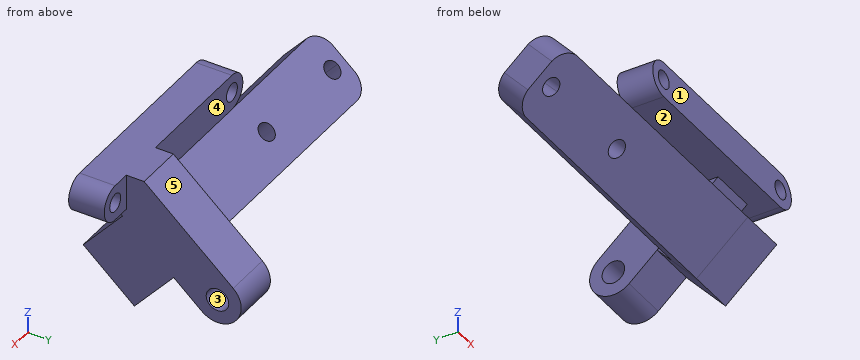
```python
from build123d import *

# Parameters (mm, degrees)
SKETCH_1_R          = 1.5
SKETCH_1_W          = 8
SKETCH_1_H          = 6
EXTRUDE_2_DEPTH     = 6
SKETCH_1_4_W        = 8
SKETCH_1_4_H        = 3
EXTRUDE_3_DEPTH     = 3
EXTRUDE_28_DEPTH    = 8
SKETCH_4_W          = 7.960549586
SKETCH_4_H          = 11.5
EXTRUDE_29_DEPTH    = 10
EXTRUDE_30_DEPTH    = 50
SKETCH_7_R          = 1.5
CUT_EXTRUDE_1_DEPTH = 10
SKETCH_8_R          = 1.9
CUT_EXTRUDE_2_DEPTH = 19


with BuildPart() as part:
    # Sketch 1 → Extrude 2 (new body)
    # profile 1 of 2: a face of its own
    with BuildSketch(Plane(origin=(0, 0, 0), x_dir=(1, 0, 0), z_dir=(0, 1, 0))):
        with BuildLine():
            Line((-38.676968887, 3), (-6.676968887, 3))
            ThreePointArc((-6.676968887, 3), (-3.676968887, 0), (-6.676968887, -3))
            Line((-6.676968887, -3), (-38.676968887, -3))
            ThreePointArc((-38.676968887, -3), (-41.676968887, 0), (-38.676968887, 3))
        make_face()
        with Locations(Location((-6.676968887, 0, 0), (0, 0, 270))):
            Circle(SKETCH_1_R, mode=Mode.SUBTRACT)
        with Locations(Location((-38.676968887, 0, 0), (0, 0, 270))):
            Circle(SKETCH_1_R, mode=Mode.SUBTRACT)
    # profile 2 of 2: a face of its own
    with BuildSketch(Plane(origin=(0, 0, 0), x_dir=(1, 0, 0), z_dir=(0, 1, 0))):
        with Locations((-13.722758256, 0)):
            Rectangle(SKETCH_1_W, SKETCH_1_H)
    extrude(amount=-EXTRUDE_2_DEPTH)

    # Sketch 1_4 → Extrude 3 (add)
    with BuildSketch(Plane(origin=(0, 0, 0), x_dir=(1, 0, 0), z_dir=(0, 1, 0))):
        with Locations((-13.722758256, -1.5)):
            Rectangle(SKETCH_1_4_W, SKETCH_1_4_H)
        with Locations((-13.722758256, 1.5)):
            Rectangle(SKETCH_1_4_W, SKETCH_1_4_H)
    extrude(amount=EXTRUDE_3_DEPTH)

    # Sketch 3 → Extrude 28 (add)
    with BuildSketch(Plane(origin=(-9.722758256, 0, 0), x_dir=(0, 0, -1), z_dir=(1, 0, 0))):
        with BuildLine():
            Line((3, -2.291502622), (16.228756555, 12.708497378))
            ThreePointArc((16.228756555, 12.708497378), (15.874507866, 18.354248689), (10.228756555, 18))
            Line((10.228756555, 18), (-3, 3))
            Line((-3, 3), (3, -2.291502622))
        make_face()
    extrude(amount=-EXTRUDE_28_DEPTH)

    # Sketch 4 → Extrude 29 (add)
    with BuildSketch(Plane(origin=(0, -2.49076751, -2.824264888), x_dir=(-1, 0, 0), z_dir=(0, -0.6614378277661491, -0.7499999999999987))):
        with Locations((13.703033049, 8.211179299)):
            Rectangle(SKETCH_4_W, SKETCH_4_H)
    extrude(amount=EXTRUDE_29_DEPTH)

    # Sketch 6 → Extrude 30 (add)
    with BuildSketch(Plane.ZY.offset(17.683307842)):
        Polygon((-19.558716996, 1.365738687), (-11.952181977, -7.259261313), (-7.452181977, -3.290634347), (-15.058716996, 5.334365653), align=None)
    extrude(amount=EXTRUDE_30_DEPTH)

    # Sketch 7 → Cut-Extrude 1 (cut)
    with BuildSketch(Plane(origin=(0, -9.105145787, -10.324264888), x_dir=(-1, 0, 0), z_dir=(0, -0.6614378277661491, -0.7499999999999987))):
        with Locations(Location((64.480624333, 8.278010001, 0), (0, 0, 90))):
            Circle(SKETCH_7_R)
        with BuildLine():
            ThreePointArc((62.982113853, 8.211179299), (64.480624333, 6.778010001), (65.979134812, 8.211179299))
            Line((65.979134812, 8.211179299), (62.982113853, 8.211179299))
        make_face()
        with BuildLine():
            Line((62.982113853, 8.211179299), (65.979134812, 8.211179299))
            ThreePointArc((65.979134812, 8.211179299), (65.980251906, 8.244586352), (65.980624333, 8.278010001))
            ThreePointArc((65.980624333, 8.278010001), (64.447200683, 9.777637575), (62.982113853, 8.211179299))
        make_face()
        with BuildLine():
            ThreePointArc((64.603588297, 13.961179299), (66.684672199, 12.962543656), (67.683307842, 10.881459754))
            Line((67.683307842, 10.881459754), (67.683307842, 13.961179299))
            Line((67.683307842, 13.961179299), (64.603588297, 13.961179299))
        make_face()
        with BuildLine():
            Line((64.603588297, 2.461179299), (67.683307842, 2.461179299))
            Line((67.683307842, 2.461179299), (67.683307842, 5.540898844))
            ThreePointArc((67.683307842, 5.540898844), (66.684672199, 3.459814942), (64.603588297, 2.461179299))
        make_face()
        with Locations(Location((46.480624333, 8.278010001, 0), (0, 0, 90))):
            Circle(SKETCH_7_R)
    extrude(amount=-CUT_EXTRUDE_1_DEPTH, mode=Mode.SUBTRACT)

    # Sketch 8 → Cut-Extrude 2 (cut)
    with BuildSketch(Plane(origin=(-9.722758256, 0, 0), x_dir=(0, 0, -1), z_dir=(1, 0, 0))):
        with Locations((13.228756555, 15.354248689)):
            Circle(SKETCH_8_R)
    extrude(amount=-CUT_EXTRUDE_2_DEPTH, mode=Mode.SUBTRACT)


solid = part.part
```
Part model, mm, in its own coordinate system. Face numbers are marked on the shaded views. A direction names the side the tool comes from. Round coordinates to 2 decimals unless told otherwise and drop trailing zeros. Loops run counter-clockwise (first coordinate to the right, second up) from the corner with the lowest first, then second, coordinate; pieces in that order, holes last. Notation, with made-up numbers: (1, 62.5) -> (27, 62.5) arc R26 cw to (27, 81.5) -> close; hole circle Ø9 at (81.25, 1). An arc over 180 degrees is marked (long way). Use a Markdown table: item, result.
1) Cut at C-C, the plane x = -17. List the corners of the cut face in (y, z).
The answers:
| item | result |
|---|---|
| outline | (-7.26, -11.95) -> (1.37, -19.56) -> (7.98, -12.06) -> (12.71, -16.23) arc R4 ccw to (18, -10.23) -> (3, 3) -> (-6, 3) -> (-6, -3) -> (-2.29, -3) -> (-0.64, -4.45) -> close; hole circle Ø3.8 at (15.35, -13.23) |
2) Pull direction Y, two halves, no side cores. Call the marked faces 1, 2 and 3: pulls with the +Y half, pulls with the -Y half, needs draft (parallel to the pull), parting line crosses it, or undercut.
The answers:
| item | result |
|---|---|
| face 1 | pulls with the -Y half |
| face 2 | needs draft |
| face 3 | undercut |
3) Tool access for the marked faces 4 and 5: list every direction of +Z, -Z, +X, -X, +Y, -Y with a clear straight run to the whole face (end or side of a thin tool).
The answers:
| item | result |
|---|---|
| face 4 | +Z, -X, +Y |
| face 5 | +Z, +X, -X, +Y |
4) Cut at B-B, the plane z = 0. List the corners of the cut face in (x, y).
The answers:
| item | result |
|---|---|
| outline | (-41.68, -6) -> (-40.18, -6) -> (-40.18, 0) -> (-41.68, 0) -> close; (-37.18, -6) -> (-8.18, -6) -> (-8.18, 0) -> (-9.72, 0) -> (-9.72, 6.4) -> (-17.72, 6.4) -> (-17.72, 0) -> (-37.18, 0) -> close; (-5.18, -6) -> (-3.68, -6) -> (-3.68, 0) -> (-5.18, 0) -> close |
5) Drop flat-ended pins along their axis: pin 1 Ø5 at (x, z) = (-35.5, -13) entering from +Y; pin 2 Ø3 at (x, z) = (-24, 1.5) entering from +Y; pin 3 Ø2 at (x, z) = (-28, -12.5) entering from +Y; pin 4 Ø2.5 at (y, z) = (15.35, -13.23) entering from +X. Give the stop position or say it passes through.
The answers:
| item | result |
|---|---|
| pin 1 | stops at y = 5.33 |
| pin 2 | stops at y = 0 |
| pin 3 | stops at y = 3.57 |
| pin 4 | passes through |
6) Cut at D-D, the plane y = 10. List the corners of the cut face in (x, z), and give its area (3 significant figures).
The answers:
| item | result |
|---|---|
| outline | (-17.72, -13.84) -> (-9.72, -13.84) -> (-9.72, -3.17) -> (-17.72, -3.17) -> close |
| area | 85.3 mm2 |
7) Cut at A-A, the plane x = -27. List the corners of the cut face in (y, z).
The answers:
| item | result |
|---|---|
| outline | (-7.26, -11.95) -> (1.37, -19.56) -> (5.33, -15.06) -> (-3.29, -7.45) -> close; (-6, -3) -> (0, -3) -> (0, 3) -> (-6, 3) -> close |
8) Probe line 1 (X direction, y = -2.85, z = 0); line 2 (X direction, y = 13.75, z = -16); line 3 (Y direction, x = -28, z = 0.5). List the from-to ranges inside material, lowest first. Write a range as [from, to].
The answers:
| item | result |
|---|---|
| line 1 | x = [-41.68, -40.18], [-37.18, -8.18], [-5.18, -3.68] |
| line 2 | x = [-17.72, -9.72] |
| line 3 | y = [-6, 0] |
